Autodesk Inventor part; units mm, degrees
ref_plane "YZ Plane" through (0, 0, 0) normal (1, 0, 0) x (0, 1, 0)
ref_plane "XZ Plane" through (0, 0, 0) normal (0, 1, 0) x (-1, 0, 0)
ref_plane "XY Plane" through (0, 0, 0) normal (0, 0, 1) x (1, 0, 0)
sketch "Sketch1" plane through (0, 0, 0) normal (0, 0, 1) x (1, 0, 0)
  line L0 (-222.9556, 663.6813) -> (246.9444, 663.6813)
  line L1 (246.9444, 663.6813) -> (246.9444, -238.0187)
  line L2 (246.9444, -238.0187) -> (-222.9556, -238.0187)
  line L3 (-222.9556, -238.0187) -> (-222.9556, 663.6813)
  point P0 (0, 0)
  dimension "d0" = 469.9
  dimension "d1" = 901.7
extrude "Board" add sketch "Sketch1" along normal blind 19.05
sketch "Sketch2" plane through (0, 0, 19.05) normal (0, 0, 1) x (1, 0, 0)
  line L0 (-222.9556, 663.6813) -> (-222.9556, -238.0187)
  line L1 (246.9444, -238.0187) -> (246.9444, 663.6813)
  line L2 (-222.9556, 69.9563) -> (246.9444, 69.9563)
  line L3 (246.9444, 69.9563) -> (246.9444, 50.9063)
  line L4 (246.9444, 50.9063) -> (-222.9556, 50.9063)
  line L5 (-222.9556, 50.9063) -> (-222.9556, 69.9563)
  line L6 (246.9444, 663.6813) -> (-222.9556, 663.6813)
  line L7 (-222.9556, -238.0187) -> (246.9444, -238.0187)
  point P0 (0, 0)
  dimension "d4" = 19.05
  dimension "d19" = 288.925
extrude "Inner Lower Shelf Dado" cut sketch "Sketch2" against normal blind 9.525 contours L2 L1 L4 L0
sketch "Sketch4" plane through (0, 0, 19.05) normal (0, 0, 1) x (1, 0, 0)
  line L0 (-222.9556, 523.9813) -> (246.9444, 523.9813)
  line L1 (246.9444, 523.9813) -> (246.9444, 504.9313)
  line L2 (246.9444, 504.9313) -> (-222.9556, 504.9313)
  line L3 (-222.9556, 504.9313) -> (-222.9556, 523.9813)
  line L4 (246.9444, 663.6813) -> (-222.9556, 663.6813)
  line L5 (246.9444, -238.0187) -> (246.9444, 663.6813)
  line L6 (-222.9556, 663.6813) -> (-222.9556, -238.0187)
  point P0 (0, 0)
  point P1 (246.9444, 69.9563)
  point P2 (-222.9556, 69.9563)
  dimension "d20" = 19.05
  dimension "d21" = 139.7
extrude "Inner Upper Shelf Dado" cut sketch "Sketch4" against normal blind 9.525 contours L0 L1 L2 L3
sketch "Sketch7" plane through (0, 0, 0) normal (0, 0, -1) x (-1, 0, 0)
  line L0 (222.9556, 663.6813) -> (-246.9444, 663.6813)
  line L1 (-246.9444, 663.6813) -> (222.9556, 663.6813)
  line L2 (222.9556, 663.6813) -> (222.9556, 650.9813)
  line L3 (222.9556, 650.9813) -> (-246.9444, 650.9813)
  line L4 (-246.9444, 650.9813) -> (-246.9444, 663.6813)
  line L5 (222.9556, -238.0187) -> (222.9556, 663.6813)
  line L6 (-246.9444, -238.0187) -> (222.9556, -238.0187)
  line L7 (222.9556, -238.0187) -> (222.9556, -228.4937)
  line L8 (222.9556, -228.4937) -> (-246.9444, -228.4937)
  line L9 (-246.9444, -228.4937) -> (-246.9444, -238.0187)
  line L10 (-246.9444, -238.0187) -> (222.9556, -238.0187)
  point P0 (0, 0)
  dimension "d32" = 12.7
  dimension "d40" = 9.525
extrude "Top and Bottom Exterior Dados" cut sketch "Sketch7" against normal blind 9.525
sketch "Sketch9" plane through (246.9444, -238.0187, 19.05) normal (1, 0, 0) x (0, 0, -1)
  line L0 (0, 901.7) -> (9.525, 901.7)
  line L1 (9.525, 901.7) -> (9.525, 0)
  line L2 (9.525, 0) -> (0, 0)
  line L3 (0, 0) -> (0, 901.7)
  line L4 (9.525, 901.7) -> (0, 901.7)
  line L5 (9.525, 0) -> (0, 0)
  line L6 (0, 0) -> (0, 742.95)
  point P0 (19.05, 238.0187)
  point P1 (0, 307.975)
  dimension "d41" = 9.525
extrude "Back Panel Notch" cut sketch "Sketch9" against normal blind 6.35
sketch "Sketch10" plane through (0, 0, 0) normal (0, 0, -1) x (-1, 0, 0)
  line L0 (-145.3444, 650.9813) -> (-107.2444, 650.9813)
  line L1 (-107.2444, 650.9813) -> (-107.2444, 630.3438)
  line L2 (-110.4194, 627.1688) -> (-142.1694, 627.1688)
  line L3 (-145.3444, 630.3438) -> (-145.3444, 650.9813)
  line L4 (-246.9444, 650.9813) -> (-246.9444, -228.4937)
  line L5 (222.9556, 650.9813) -> (-246.9444, 650.9813)
  line L6 (95.9556, 650.9813) -> (134.0556, 650.9813)
  line L7 (134.0556, 650.9813) -> (134.0556, 630.3438)
  line L8 (130.8806, 627.1688) -> (99.1306, 627.1688)
  line L9 (95.9556, 630.3438) -> (95.9556, 650.9813)
  arc A0 (-145.3444, 630.3438) -> (-142.1694, 627.1688) centre (-142.1694, 630.3438) ccw
  arc A1 (-110.4194, 627.1688) -> (-107.2444, 630.3438) centre (-110.4194, 630.3438) ccw
  arc A2 (95.9556, 630.3438) -> (99.1306, 627.1688) centre (99.1306, 630.3438) ccw
  arc A3 (130.8806, 627.1688) -> (134.0556, 630.3438) centre (130.8806, 630.3438) ccw
  point P0 (0, 0)
  point P1 (-107.2444, 627.1688)
  point P2 (-145.3444, 627.1688)
  point P3 (134.0556, 627.1688)
  point P4 (95.9556, 627.1688)
  dimension "d44" = 38.1
  dimension "d45" = 23.8125
  dimension "d46" = 101.6
  dimension "d47" = 38.1
  dimension "d48" = 23.8125
  dimension "d49" = 203.2
  dimension "d50" = 3.175
extrude "Top Hinge Notches" cut sketch "Sketch10" against normal blind 3.175
sketch "Sketch12" plane through (-222.9556, -238.0187, 19.05) normal (-1, 0, 0) x (0, 0, 1)
  line L0 (-9.525, 9.525) -> (-9.525, 0)
  line L1 (0, 901.7) -> (0, 0)
  line L2 (-9.525, 0) -> (0, 0)
  line L3 (0, 0) -> (0, 9.525)
  line L4 (0, 9.525) -> (-9.525, 9.525)
  line L5 (-9.525, 9.525) -> (-9.525, 0)
  line L6 (-19.05, 9.525) -> (-9.525, 9.525)
  point P0 (-19.05, 238.0187)
  point P1 (0, 288.925)
extrude "Front notch to cover dado" cut sketch "Sketch12" against normal blind 6.35
sketch "Sketch3" plane through (0, 0, 19.05) normal (0, 0, 1) x (1, 0, 0)
  line L0 (240.5944, -133.2437) -> (-95.9556, -133.2437)
  line L1 (-95.9556, -133.2437) -> (-95.9556, -139.5937)
  line L2 (-95.9556, -139.5937) -> (240.5944, -139.5937)
  line L3 (240.5944, -139.5937) -> (240.5944, -133.2437)
  line L4 (-222.9556, -238.0187) -> (246.9444, -238.0187)
  line L5 (259.6444, -37.9937) -> (-95.9556, -37.9937)
  line L6 (-95.9556, -37.9937) -> (-95.9556, -44.3437)
  line L7 (-95.9556, -44.3437) -> (259.6444, -44.3437)
  line L8 (259.6444, -44.3437) -> (259.6444, -37.9937)
  line L9 (-222.9556, 663.6813) -> (-222.9556, -238.0187)
  line L10 (246.9444, 50.9063) -> (-222.9556, 50.9063)
  line L11 (246.9444, -228.4937) -> (240.5944, -228.4937)
  point P0 (0, 0)
  dimension "d9" = 6.35
  dimension "d14" = 6.35
  dimension "d17" = 88.9
  dimension "d26" = 127
  dimension "d67" = 88.9
extrude "Inner Wine Rack Dados" cut sketch "Sketch3" against normal blind 6.35
sketch "Sketch8" plane through (0, 0, 19.05) normal (0, 0, 1) x (1, 0, 0)
  line L0 (246.9444, 50.9063) -> (-222.9556, 50.9063)
  line L1 (132.6444, -238.0187) -> (138.9944, -238.0187)
  line L2 (138.9944, -238.0187) -> (138.9944, 50.9063)
  line L3 (138.9944, 50.9063) -> (132.6444, 50.9063)
  line L4 (132.6444, 50.9063) -> (132.6444, -238.0187)
  line L5 (-95.9556, -139.5937) -> (-95.9556, -133.2437)
  line L6 (-222.9556, -238.0187) -> (246.9444, -238.0187)
  point P0 (0, 0)
  dimension "d35" = 6.35
  dimension "d36" = 228.6
extrude "Vertical Wine Bottle False Back" cut sketch "Sketch8" against normal blind 9.525
sketch "Sketch13" plane through (0, 0, 9.525) normal (0, 0, -1) x (-1, 0, 0)
  line L0 (-246.9444, 650.9813) -> (-246.9444, -228.4937)
  line L1 (216.6056, -238.0187) -> (-240.5944, -238.0187)
  line L2 (-246.9444, -228.4937) -> (-227.8944, -228.4937)
  line L3 (-227.8944, -228.4937) -> (-227.8944, -238.0187)
  line L4 (-227.8944, -238.0187) -> (-246.9444, -238.0187)
  line L5 (-246.9444, -238.0187) -> (-246.9444, -228.4937)
  point P0 (0, 0)
  point P1 (-138.9944, -238.0187)
  dimension "d64" = 19.05
extrude "Rear notch for bottom runner" cut sketch "Sketch13" against normal blind 19.05
equation "\"d6\" = 0.5 * d2"
equation "\"d22\" = 0.5 * d2"
equation "\"d49\" = 2 * d46"
equation "\"d37\" = 0.5 * d2"
properties part number "Left Side"
Source: CAD feature listing. Evaluate the final solid. Frame: model axes, mm. A direction names the side the tool comes from. Coordinates: 2 decimals unless noted, no trailing zeros. Loops run counter-clockwise (first coordinate to the right, second up) from the corner with the lowest first, then second, coordinate; pieces in that order, holes last. Notation, with made-up numbers: M 13,39.5 L 23,39.5 A17 cw 23,59.5 Z; hole C 7.5,-14.75 d2. An arc over 180 degrees is marked long. Answer in a Markdown table with one row per item.
Q1. Section D-D on x = -41.5. Return the cut outline in (y, z) (3 decimals).
Answers below:
| item | result |
|---|---|
| outline | M -238.019,9.525 L -228.494,9.525 L -228.494,0 L 650.981,0 L 650.981,9.525 L 663.681,9.525 L 663.681,19.05 L 523.981,19.05 L 523.981,9.525 L 504.931,9.525 L 504.931,19.05 L 69.956,19.05 L 69.956,9.525 L 50.906,9.525 L 50.906,19.05 L -37.994,19.05 L -37.994,12.7 L -44.344,12.7 L -44.344,19.05 L -133.244,19.05 L -133.244,12.7 L -139.594,12.7 L -139.594,19.05 L -238.019,19.05 Z |
Q2. Ray query, probe 1 along Y at (x, z) = (-33, 13.5); probe 2 along Y at (x, z) = (-31, 11.75); probe 3 along X at (y, z) = (-78.5, 14.25). Return the intervals inside material, ascending. Write a range as from..to.
Answers below:
| item | result |
|---|---|
| probe 1 | y = -238.02..-139.59, -133.24..-44.34, -37.99..50.91, 69.96..504.93, 523.98..663.68 |
| probe 2 | y = -238.02..50.91, 69.96..504.93, 523.98..663.68 |
| probe 3 | x = -222.96..132.64, 138.99..240.59 |
Q3. Section A-A on x = -180. Return the cut outline in (y, z) (3 decimals).
Answers below:
| item | result |
|---|---|
| outline | M -238.019,9.525 L -228.494,9.525 L -228.494,0 L 650.981,0 L 650.981,9.525 L 663.681,9.525 L 663.681,19.05 L 523.981,19.05 L 523.981,9.525 L 504.931,9.525 L 504.931,19.05 L 69.956,19.05 L 69.956,9.525 L 50.906,9.525 L 50.906,19.05 L -238.019,19.05 Z |
Q4. Draft query along Y for faces 1 (the flat face through (48, 506, 9.525)), 2 (the flat face through (-222.956, 211, 9)). Return one class per face: pulls with the +Y half, pulls with the -Y half, needs draft (parallel to the pull), parting line crosses it, or undercut.
Answers below:
| item | result |
|---|---|
| face 1 | undercut |
| face 2 | needs draft |
Q5. First-contact query: pin 1 (3 mm diameter, centred on y = -41, z = 16.5, fed in from +X); pin 2 (7 mm diameter, centred on x = -119, y = 634.5, fed in from -Z) (3 decimals); pin 3 (5 mm diameter, centred on x = 38.5, y = -41.5, fed in from +Z). Flat tips, straight axial feed; report the tip coordinate or a pass-through.
Answers below:
| item | result |
|---|---|
| pin 1 | stops at x = -95.96 |
| pin 2 | stops at z = 3.175 |
| pin 3 | stops at z = 12.7 |
Q6. Section C-C on x = -116.5. Return the cut outline in (y, z) (3 decimals).
Answers below:
| item | result |
|---|---|
| outline | M -238.019,9.525 L -228.494,9.525 L -228.494,0 L 627.169,0 L 627.169,3.175 L 650.981,3.175 L 650.981,9.525 L 663.681,9.525 L 663.681,19.05 L 523.981,19.05 L 523.981,9.525 L 504.931,9.525 L 504.931,19.05 L 69.956,19.05 L 69.956,9.525 L 50.906,9.525 L 50.906,19.05 L -238.019,19.05 Z |
Q7. Section B-B on z = 6.5. Return the cut outline in (x, y), plus the area to 3 significant figures.
Answers below:
| item | result |
|---|---|
| outline | M -222.96,-228.49 L 246.94,-228.49 L 246.94,650.98 L -222.96,650.98 Z |
| area | 413,000 mm^2 |
Q8. Set-up query: faces 3 (the flat face through (127, 639, 3.175)), 4 (the flat face through (-48, -92, 19.05)). Return all of +Z, -Z, +X, -X, +Y, -Y with unobstructed straight access to the full face (end or side cutting, diameter ignored); none if empty.
Answers below:
| item | result |
|---|---|
| face 3 | -Z, +Y |
| face 4 | +Z, +X, -X, +Y, -Y |
